from build123d import *

# Parameters (mm, degrees)
SKETCH1_R           = 0.375
SKETCH1_R_2         = 0.75
BOSS_EXTRUDE1_DEPTH = 0.5
SKETCH1_2_R         = 0.375
BOSS_EXTRUDE2_DEPTH = 2.5
SKETCH1_3_R         = 0.75
BOSS_EXTRUDE3_DEPTH = 3.3
SKETCH2_R           = 0.375
SKETCH2_R_2         = 0.75
BOSS_EXTRUDE4_DEPTH = 0.5


with BuildPart() as part:
    # Sketch1 → Boss-Extrude1 (new body, symmetric)
    with BuildSketch(Plane.XY):
        with BuildLine():
            Line((-10.217126409, 0.549866302), (10.182951984, 0.999756913))
            ThreePointArc((10.182951984, 0.999756913), (11.205, 0), (10.182951984, -0.999756913))
            Line((10.182951984, -0.999756913), (-10.217126409, -0.549866302))
            ThreePointArc((-10.217126409, -0.549866302), (-10.755, 0), (-10.217126409, 0.549866302))
        make_face()
        with Locations((-10.205, 0)):
            Circle(SKETCH1_R, mode=Mode.SUBTRACT)
        with Locations((10.205, 0)):
            Circle(SKETCH1_R_2, mode=Mode.SUBTRACT)
    extrude(amount=BOSS_EXTRUDE1_DEPTH, both=True)

    # Sketch1<2> → Boss-Extrude2 (add)
    with BuildSketch(Plane.XY):
        with Locations((-10.205, 0)):
            Circle(SKETCH1_2_R)
    extrude(amount=BOSS_EXTRUDE2_DEPTH)

    # Sketch1<3> → Boss-Extrude3 (add)
    with BuildSketch(Plane.XY):
        with Locations((10.205, 0)):
            Circle(SKETCH1_3_R)
    extrude(amount=BOSS_EXTRUDE3_DEPTH)

    # Sketch2 → Boss-Extrude4 (add)
    with BuildSketch(Plane(origin=(0, 0, 0), x_dir=(-1, 0, 0), z_dir=(0, 0, -1))):
        with Locations((10.205, 0)):
            Circle(SKETCH2_R)
        with Locations((-10.205, 0)):
            Circle(SKETCH2_R_2)
    extrude(amount=BOSS_EXTRUDE4_DEPTH)


solid = part.part
Source: CAD feature listing. Evaluate the final solid. Frame: model axes, mm. A direction names the side the tool comes from. Round coordinates to 2 decimals unless told otherwise and drop trailing zeros. Loops run counter-clockwise (first coordinate to the right, second up) from the corner with the lowest first, then second, coordinate; pieces in that order, holes last. Notation, with made-up numbers: (34, 42.5) -> (70, 42.5) arc R33 cw to (70, 71.5) -> close; hole circle Ø7 at (34, -14.5). An arc over 180 degrees is marked (long way). Answer as a JSON object with one key per item and string values. Group by question number.
Q1. Section query A-A (y = 0). Output: boundary loops of the cut face in (x, z) (3 decimals), plus the area to 3 significant figures.
Q2. Ray query, line 1 (X direction, y = 0.05, z = 2.45); line 2 (Z direction, x = 8.5, y = 0.7); line 3 (X direction, y = 0.1, z = 3). Return the intervals inside material, ascending. Write a range as from..to.
Q3. Section query B-B (z = 1.6). Output: boundary loops of the cut face in (x, y) (3 decimals).
Q4. Section query D-D (x = -1.5). Output: boundary loops of the cut face in (y, z), plus the area to 3 significant figures.
Q5. Contact query for flat-ended pins moving along their axis: P1, Ø0.6, axis at x = 1, y = 0.5, coming from the +Z side; P2, Ø0.6, axis at x = -10.5, y = 0, coming from the +Z side. Output: stop coordinate, or through.
Q6. Section query C-C (z = 3). Output: boundary loops of the cut face in (x, y) (3 decimals).
Q7. Mould query, pull axis X, two halves, no side actions, for faces 1 (the flat face through (3, 0, -0.5)), 2 (the cylindrical face through (-10.755, -0.012, 0.007)), 3 (the flat face through (0, 0, 0.5)). Classes: pulls with the +X half, pulls with the -X half, needs draft (parallel to the pull), parting line crosses it, or undercut.
Q8. Access query for faces 4 (the cylindrical face through (10.92, 0.23, 1.88)), 5 (the flat face through (10, 0, 3.3)). Directions: +Z, -Z, +X, -X, +Y, -Y. A direction counts if a zero-diameter tool reaches every point of the face in a straight line with its end or side. Return the directions, or none.
Completed:
{
 "1": {"outline": "(-10.755, -0.5) -> (11.205, -0.5) -> (11.205, 0.5) -> (10.955, 0.5) -> (10.955, 3.3) -> (9.455, 3.3) -> (9.455, 0.5) -> (-9.83, 0.5) -> (-9.83, 2.5) -> (-10.58, 2.5) -> (-10.58, 0.5) -> (-10.755, 0.5) -> close", "area": "27.7 mm²"},
 "2": {"line 1": "-10.58..-9.83, 9.46..10.95", "line 2": "-0.5..0.5", "line 3": "9.46..10.95"},
 "3": {"outline": "circle Ø0.75 at (-10.205, 0); circle Ø1.5 at (10.205, 0)"},
 "4": {"outline": "(-0.74, -0.5) -> (0.74, -0.5) -> (0.74, 0.5) -> (-0.74, 0.5) -> close", "area": "1.48 mm²"},
 "5": {"P1": "z = 0.5", "P2": "z = 2.5"},
 "6": {"outline": "circle Ø1.5 at (10.205, 0)"},
 "7": {"face 1": "needs draft", "face 2": "pulls with the -X half", "face 3": "undercut"},
 "8": {"face 4": "+Z", "face 5": "+Z, +X, -X, +Y, -Y"}
}
